Read the model definition and answer for the solid it produces. Units are mm, in the model's axes. Face numbers are marked on the shaded views. A direction names the side the tool comes from. Coordinates: 2 decimals unless noted, no trailing zeros. Write each loop counter-clockwise with the first axis right and the second up, starting at its lowest first coordinate (ties: lowest second). Pieces come first, ordered by that corner, then holes. Notation, with made-up numbers: (-15, 75.25) -> (-7, 75.25) arc R22 cw to (-7, 95.25) -> close; hole circle Ø11 at (11, -26). An arc over 180 degrees is marked (long way). Use CSV: the item, a comma, the result in double quotes.
from build123d import *

# Parameters (mm, degrees)
BOSS_EXTRUDE1_DEPTH     = 2
SKETCH1_4_R             = 1.5
BOSS_EXTRUDE2_DEPTH     = 19
BOSS_EXTRUDE2_2_DEPTH   = 19
BOSS_EXTRUDE2_3_DEPTH   = 19
BOSS_EXTRUDE2_4_DEPTH   = 19
BOSS_EXTRUDE2_5_DEPTH   = 19
BOSS_EXTRUDE2_6_DEPTH   = 19
SKETCH1_5_R             = 1.5
BOSS_EXTRUDE3_DEPTH     = 20
BOSS_EXTRUDE4_DEPTH     = 22
SKETCH2_W               = 23
SKETCH2_H               = 8
SKETCH2_W_2             = 13.5
SKETCH2_H_2             = 13.3
CUT_EXTRUDE1_DEPTH      = 3
SKETCH3_W               = 20
SKETCH3_H               = 12
SKETCH3_W_2             = 33
CUT_EXTRUDE2_DEPTH      = 3
SKETCH4_W               = 12
SKETCH4_H               = 7.5
CUT_EXTRUDE3_DEPTH      = 3
CUT_EXTRUDE4_DEPTH      = 1
CUT_EXTRUDE4_DEPTH_BACK = 2
SKETCH6_W               = 20
SKETCH6_H               = 8
SKETCH6_W_2             = 33
CUT_EXTRUDE5_DEPTH      = 2
CUT_EXTRUDE6_DEPTH      = 1
CUT_EXTRUDE6_DEPTH_BACK = 2


with BuildPart() as part:
    # Sketch1 → Boss-Extrude1 (new body)
    with BuildSketch(Plane(origin=(0, 0, 0), x_dir=(1, 0, 0), z_dir=(0, 1, 0))):
        with BuildLine():
            ThreePointArc((86, 27), (87.318019485, 23.818019485), (90.5, 22.5))
            Line((90.5, 22.5), (93, 22.5))
            Line((93, 22.5), (93, -22.5))
            Line((93, -22.5), (90.5, -22.5))
            ThreePointArc((90.5, -22.5), (87.318019485, -23.818019485), (86, -27))
            Line((86, -27), (86, -29.5))
            Line((86, -29.5), (4.5, -29.5))
            Line((4.5, -29.5), (4.5, -27))
            ThreePointArc((4.5, -27), (0, -22.5), (-4.5, -27))
            Line((-4.5, -27), (-4.5, -29.5))
            Line((-4.5, -29.5), (-86, -29.5))
            Line((-86, -29.5), (-86, -27))
            ThreePointArc((-86, -27), (-87.318019485, -23.818019485), (-90.5, -22.5))
            Line((-90.5, -22.5), (-93, -22.5))
            Line((-93, -22.5), (-93, 22.5))
            Line((-93, 22.5), (-90.5, 22.5))
            ThreePointArc((-90.5, 22.5), (-87.318019485, 23.818019485), (-86, 27))
            Line((-86, 27), (-86, 29.5))
            Line((-86, 29.5), (-4.5, 29.5))
            Line((-4.5, 29.5), (-4.5, 27))
            ThreePointArc((-4.5, 27), (0, 22.5), (4.5, 27))
            Line((4.5, 27), (4.5, 29.5))
            Line((4.5, 29.5), (86, 29.5))
            Line((86, 29.5), (86, 27))
        make_face()
    extrude(amount=BOSS_EXTRUDE1_DEPTH)



with BuildPart() as body_2:
    # Sketch1<4> → Boss-Extrude2 (new body)
    with BuildSketch(Plane(origin=(0, 0, 0), x_dir=(1, 0, 0), z_dir=(0, 1, 0))):
        with Locations((90.5, 27)):
            Circle(SKETCH1_4_R)
    extrude(amount=BOSS_EXTRUDE2_DEPTH)



with BuildPart() as body_3:
    # Sketch1<4> → Boss-Extrude2 2 (new body)
    with BuildSketch(Plane(origin=(0, 0, 0), x_dir=(1, 0, 0), z_dir=(0, 1, 0))):
        with Locations((90.5, -27)):
            Circle(SKETCH1_4_R)
    extrude(amount=BOSS_EXTRUDE2_2_DEPTH)


with BuildPart() as body_4:
    # Sketch1<4> → Boss-Extrude2 3 (new body)
    with BuildSketch(Plane(origin=(0, 0, 0), x_dir=(1, 0, 0), z_dir=(0, 1, 0))):
        with Locations((0, -27)):
            Circle(SKETCH1_4_R)
    extrude(amount=BOSS_EXTRUDE2_3_DEPTH)


with BuildPart() as body_5:
    # Sketch1<4> → Boss-Extrude2 4 (new body)
    with BuildSketch(Plane(origin=(0, 0, 0), x_dir=(1, 0, 0), z_dir=(0, 1, 0))):
        with Locations((0, 27)):
            Circle(SKETCH1_4_R)
    extrude(amount=BOSS_EXTRUDE2_4_DEPTH)


with BuildPart() as body_6:
    # Sketch1<4> → Boss-Extrude2 5 (new body)
    with BuildSketch(Plane(origin=(0, 0, 0), x_dir=(1, 0, 0), z_dir=(0, 1, 0))):
        with Locations((-90.5, 27)):
            Circle(SKETCH1_4_R)
    extrude(amount=BOSS_EXTRUDE2_5_DEPTH)


with BuildPart() as body_7:
    # Sketch1<4> → Boss-Extrude2 6 (new body)
    with BuildSketch(Plane(origin=(0, 0, 0), x_dir=(1, 0, 0), z_dir=(0, 1, 0))):
        with Locations((-90.5, -27)):
            Circle(SKETCH1_4_R)
    extrude(amount=BOSS_EXTRUDE2_6_DEPTH)


with BuildPart() as body_2_1:
    add(body_2.part)

    add(body_3.part)  # Boss-Extrude3 merges body 3

    add(body_4.part)  # Boss-Extrude3 merges body 4

    add(body_5.part)  # Boss-Extrude3 merges body 5

    add(body_6.part)  # Boss-Extrude3 merges body 6

    add(body_7.part)  # Boss-Extrude3 merges body 7
    # Sketch1<5> → Boss-Extrude3 (add)
    with BuildSketch(Plane(origin=(0, 0, 0), x_dir=(1, 0, 0), z_dir=(0, 1, 0))):
        Polygon((93.5, 27), (92, 24.401923789), (89, 24.401923789), (87.5, 27), (89, 29.598076211), (92, 29.598076211), align=None)
        with Locations((90.5, 27)):
            Circle(SKETCH1_5_R, mode=Mode.SUBTRACT)
        Polygon((89, -29.598076211), (92, -29.598076211), (93.5, -27), (92, -24.401923789), (89, -24.401923789), (87.5, -27), align=None)
        with Locations((90.5, -27)):
            Circle(SKETCH1_5_R, mode=Mode.SUBTRACT)
        Polygon((3, -27), (1.5, -29.598076211), (-1.5, -29.598076211), (-3, -27), (-1.5, -24.401923789), (1.5, -24.401923789), align=None)
        with Locations((0, -27)):
            Circle(SKETCH1_5_R, mode=Mode.SUBTRACT)
        Polygon((-1.5, 24.401923789), (1.5, 24.401923789), (3, 27), (1.5, 29.598076211), (-1.5, 29.598076211), (-3, 27), align=None)
        with Locations((0, 27)):
            Circle(SKETCH1_5_R, mode=Mode.SUBTRACT)
        Polygon((-93.5, -27), (-92, -24.401923789), (-89, -24.401923789), (-87.5, -27), (-89, -29.598076211), (-92, -29.598076211), align=None)
        with Locations((-90.5, -27)):
            Circle(SKETCH1_5_R, mode=Mode.SUBTRACT)
        Polygon((-89, 29.598076211), (-92, 29.598076211), (-93.5, 27), (-92, 24.401923789), (-89, 24.401923789), (-87.5, 27), align=None)
        with Locations((-90.5, 27)):
            Circle(SKETCH1_5_R, mode=Mode.SUBTRACT)
    extrude(amount=BOSS_EXTRUDE3_DEPTH)


with BuildPart() as part_1:
    add(part.part)

    add(body_2_1.part)  # Boss-Extrude4 merges body 2
    # Sketch1<6> → Boss-Extrude4 (add)
    with BuildSketch(Plane(origin=(0, 0, 0), x_dir=(1, 0, 0), z_dir=(0, 1, 0))):
        Polygon((-95, -22.5), (-95, -31.5), (-86, -31.5), (86, -31.5), (95, -31.5), (95, -22.5), (95, 22.5), (95, 31.5), (86, 31.5), (4.5, 31.5), (-4.5, 31.5), (-86, 31.5), (-95, 31.5), (-95, 22.5), align=None)
        Polygon((-89, -29.598076211), (-92, -29.598076211), (-93.5, -27), (-92, -24.401923789), (-89, -24.401923789), (-87.5, -27), align=None, mode=Mode.SUBTRACT)
        Polygon((-1.5, -24.401923789), (1.5, -24.401923789), (3, -27), (1.5, -29.598076211), (-1.5, -29.598076211), (-3, -27), align=None, mode=Mode.SUBTRACT)
        Polygon((92, -29.598076211), (89, -29.598076211), (87.5, -27), (89, -24.401923789), (92, -24.401923789), (93.5, -27), align=None, mode=Mode.SUBTRACT)
        Polygon((-92, 24.401923789), (-93.5, 27), (-92, 29.598076211), (-89, 29.598076211), (-87.5, 27), (-89, 24.401923789), align=None, mode=Mode.SUBTRACT)
        Polygon((1.5, 29.598076211), (3, 27), (1.5, 24.401923789), (-1.5, 24.401923789), (-3, 27), (-1.5, 29.598076211), align=None, mode=Mode.SUBTRACT)
        with BuildLine():
            Line((-93, -22.5), (-93, 22.5))
            Line((-93, 22.5), (-90.5, 22.5))
            ThreePointArc((-90.5, 22.5), (-87.318019485, 23.818019485), (-86, 27))
            Line((-86, 27), (-86, 29.5))
            Line((-86, 29.5), (-4.5, 29.5))
            Line((-4.5, 29.5), (-4.5, 27))
            ThreePointArc((-4.5, 27), (0, 22.5), (4.5, 27))
            Line((4.5, 27), (4.5, 29.5))
            Line((4.5, 29.5), (86, 29.5))
            Line((86, 29.5), (86, 27))
            ThreePointArc((86, 27), (87.318019485, 23.818019485), (90.5, 22.5))
            Line((90.5, 22.5), (93, 22.5))
            Line((93, 22.5), (93, -22.5))
            Line((93, -22.5), (90.5, -22.5))
            ThreePointArc((90.5, -22.5), (87.318019485, -23.818019485), (86, -27))
            Line((86, -27), (86, -29.5))
            Line((86, -29.5), (4.5, -29.5))
            Line((4.5, -29.5), (4.5, -27))
            ThreePointArc((4.5, -27), (0, -22.5), (-4.5, -27))
            Line((-4.5, -27), (-4.5, -29.5))
            Line((-4.5, -29.5), (-86, -29.5))
            Line((-86, -29.5), (-86, -27))
            ThreePointArc((-86, -27), (-87.318019485, -23.818019485), (-90.5, -22.5))
            Line((-90.5, -22.5), (-93, -22.5))
        make_face(mode=Mode.SUBTRACT)
        Polygon((89, 29.598076211), (92, 29.598076211), (93.5, 27), (92, 24.401923789), (89, 24.401923789), (87.5, 27), align=None, mode=Mode.SUBTRACT)
    extrude(amount=BOSS_EXTRUDE4_DEPTH)

    # Sketch2 → Cut-Extrude1 (cut)
    with BuildSketch(Plane(origin=(95, 0, 0), x_dir=(0, 0, -1), z_dir=(1, 0, 0))):
        with Locations((-10, 6)):
            Rectangle(SKETCH2_W, SKETCH2_H)
        with Locations((14.75, 8.65)):
            Rectangle(SKETCH2_W_2, SKETCH2_H_2)
    extrude(amount=-CUT_EXTRUDE1_DEPTH, mode=Mode.SUBTRACT)

    # Sketch3 → Cut-Extrude2 (cut)
    with BuildSketch(Plane(origin=(0, 0, -31.5), x_dir=(-1, 0, 0), z_dir=(0, 0, -1))):
        with Locations((-65, 8)):
            Rectangle(SKETCH3_W, SKETCH3_H)
        with Locations((51.5, 8)):
            Rectangle(SKETCH3_W_2, SKETCH3_H)
    extrude(amount=-CUT_EXTRUDE2_DEPTH, mode=Mode.SUBTRACT)

    # Sketch4 → Cut-Extrude3 (cut)
    with BuildSketch(Plane.ZY.offset(95)):
        with Locations((-9.5, 5.75)):
            Rectangle(SKETCH4_W, SKETCH4_H)
        with Locations((9.5, 5.75)):
            Rectangle(SKETCH4_W, SKETCH4_H)
    extrude(amount=-CUT_EXTRUDE3_DEPTH, mode=Mode.SUBTRACT)

    # Sketch5 → Cut-Extrude4 (cut, two sides)
    with BuildSketch(Plane(origin=(95, 0, 0), x_dir=(0, 0, -1), z_dir=(1, 0, 0))) as cut_extrude4_sk:
        Polygon((-21.5, 22), (-21.5, 10), (1.5, 10), (8, 10), (8, 15.3), (21.5, 15.3), (21.5, 22), align=None)
    extrude(amount=CUT_EXTRUDE4_DEPTH, mode=Mode.SUBTRACT)
    extrude(cut_extrude4_sk.sketch, amount=-CUT_EXTRUDE4_DEPTH_BACK, mode=Mode.SUBTRACT)

    # Sketch6 → Cut-Extrude5 (cut)
    with BuildSketch(Plane(origin=(0, 0, -31.5), x_dir=(-1, 0, 0), z_dir=(0, 0, -1))):
        with Locations((-65, 18)):
            Rectangle(SKETCH6_W, SKETCH6_H)
        with Locations((51.5, 18)):
            Rectangle(SKETCH6_W_2, SKETCH6_H)
    extrude(amount=-CUT_EXTRUDE5_DEPTH, mode=Mode.SUBTRACT)

    # Sketch7 → Cut-Extrude6 (cut, two sides)
    with BuildSketch(Plane.ZY.offset(95)) as cut_extrude6_sk:
        Polygon((-15.5, 22), (-15.5, 9.5), (-3.5, 9.5), (3.5, 9.5), (15.5, 9.5), (15.5, 22), align=None)
    extrude(amount=CUT_EXTRUDE6_DEPTH, mode=Mode.SUBTRACT)
    extrude(cut_extrude6_sk.sketch, amount=-CUT_EXTRUDE6_DEPTH_BACK, mode=Mode.SUBTRACT)


solid = part_1.part
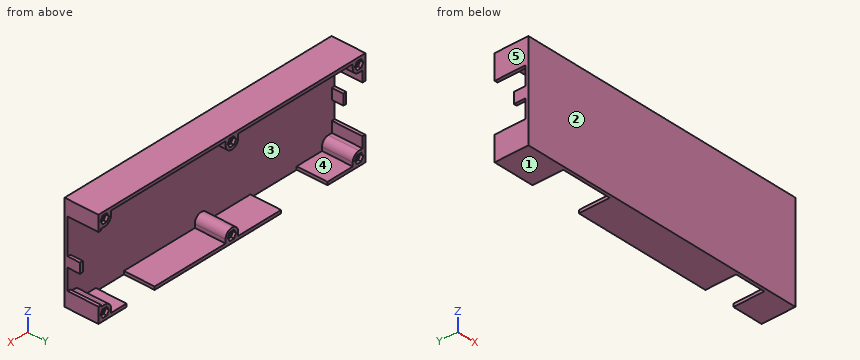
1. A cutting plane is placed at D-D (x = -55). Give the vertices of the cut face in (y, z), and give its area (3 significant figures).
Solutions:
outline,"(0, -31.5) -> (2, -31.5) -> (2, 29.5) -> (22, 29.5) -> (22, 31.5) -> (0, 31.5) -> close"
area,"166 mm^2"
2. For a pull along Z with two mould halves and no side action, classify the marked faces 1, 2 and 3 as pulls with the +Z half, pulls with the -Z half, needs draft (parallel to the pull), parting line crosses it, or undercut.
Solutions:
face 1,"pulls with the -Z half"
face 2,"needs draft"
face 3,"undercut"
3. A tool of negligible diameter and unlimited length cuts with its end or side. For the marked faces 4 and 5, from which of +Z, -Z, +X, -X, +Y, -Y can it reach the whole face along a straight path? Write none if from no direction.
Solutions:
face 4,"+Y"
face 5,"+Z, -Z, -X, +Y, -Y"
4. A cutting plane is placed at C-C (z = 9.5). Give the vertices of the cut face in (x, y).
Solutions:
outline,"(-95, 0) -> (95, 0) -> (95, 2) -> (-95, 2) -> close"
5. A cutting plane is placed at A-A (x = -76). Give the vertices of the cut face in (y, z), and give its area (3 significant figures).
Solutions:
outline,"(0, -31.5) -> (22, -31.5) -> (22, -29.5) -> (2, -29.5) -> (2, 29.5) -> (22, 29.5) -> (22, 31.5) -> (0, 31.5) -> close"
area,"206 mm^2"
6. Find the intervals of material crossed by line 1 along X through (y, z) = (19.7, 27); line 2 along Z through (x, y) = (0, 19.35); line 3 along Z through (x, y) = (-78, 17.5), in increasing order.
Solutions:
line 1,"x = -95 to -92, -89 to -86, -4.5 to -1.5, 1.5 to 4.5, 86 to 89, 92 to 95"
line 2,"z = -31.5 to -28.5, -25.5 to -22.5, 22.5 to 25.5, 28.5 to 31.5"
line 3,"z = -31.5 to -29.5, 29.5 to 31.5"
7. A cutting plane is placed at B-B (y = 4.5). Give the number of separate pieces and of enclosed holes in the cut face, and give its area (3 significant figures).
Solutions:
separate pieces,"6"
enclosed holes,"0"
area,"1,060 mm^2"
8. Each of these flat-tipped pins is pushed along its axis until it touches: pin 1 Ø2 at (x, z) = (94.5, -5) entering from +Y; pin 2 Ø4 at (x, z) = (0, 27) entering from +Y; pin 3 Ø1.5 at (y, z) = (14, -17.5) entering from +X. Where does it stop, or does it pass through?
Solutions:
pin 1,"stops at y = 10"
pin 2,"stops at y = 20"
pin 3,"stops at x = -93"
